from build123d import *

# Parameters (mm, degrees)
BOSS_EXTRUDE1_DEPTH     = 190
SKETCH2_W               = 50
SKETCH2_H               = 20
CUT_EXTRUDE1_DEPTH      = 50
SKETCH3_W               = 50
SKETCH3_H               = 80
CUT_EXTRUDE2_DEPTH      = 50
SKETCH4_W               = 50
SKETCH4_H               = 35
CUT_EXTRUDE4_DEPTH      = 50
SKETCH9_W               = 15
SKETCH9_H               = 5
BOSS_EXTRUDE4_DEPTH     = 5
SKETCH5_R               = 1
CUT_EXTRUDE5_DEPTH      = 10
CUT_EXTRUDE6_DEPTH      = 100
CUT_EXTRUDE6_DEPTH_BACK = 10
SKETCH6_R               = 1
FILLET1_R               = 1
FILLET2_R               = 2


with BuildPart() as part:
    # Sketch1 → Boss-Extrude1 (new body)
    with BuildSketch(Plane.XY):
        Polygon((-5.73630137, 0.530821918), (9.26369863, 0.530821918), (9.26369863, -1.469178082), (59.26369863, -1.469178082), (59.26369863, 0.530821918), (74.26369863, 0.530821918), (74.26369863, -4.469178082), (69.26369863, -4.469178082), (69.26369863, -7.469178082), (66.26369863, -7.469178082), (66.26369863, -4.469178082), (2.26369863, -4.469178082), (2.26369863, -7.469178082), (-0.73630137, -7.469178082), (-0.73630137, -4.469178082), (-5.73630137, -4.469178082), align=None)
    extrude(amount=BOSS_EXTRUDE1_DEPTH)

    # Sketch2 → Cut-Extrude1 (cut)
    with BuildSketch(Plane(origin=(0, -1.469178082, 0), x_dir=(1, 0, 0), z_dir=(0, 1, 0))):
        with Locations((34.26369863, -10)):
            Rectangle(SKETCH2_W, SKETCH2_H)
        with Locations((34.26369863, -190)):
            Rectangle(SKETCH2_W, SKETCH2_H)
    extrude(amount=-CUT_EXTRUDE1_DEPTH, mode=Mode.SUBTRACT)

    # Sketch3 → Cut-Extrude2 (cut)
    with BuildSketch(Plane(origin=(0, -1.469178082, 0), x_dir=(1, 0, 0), z_dir=(0, 1, 0))):
        with Locations((34.26369863, -75)):
            Rectangle(SKETCH3_W, SKETCH3_H)
    extrude(amount=-CUT_EXTRUDE2_DEPTH, mode=Mode.SUBTRACT)

    # Sketch4 → Cut-Extrude4 (cut)
    with BuildSketch(Plane(origin=(0, -1.469178082, 0), x_dir=(1, 0, 0), z_dir=(0, 1, 0))):
        with Locations((34.26369863, -147.5)):
            Rectangle(SKETCH4_W, SKETCH4_H)
    extrude(amount=-CUT_EXTRUDE4_DEPTH, mode=Mode.SUBTRACT)

    # Sketch9 → Boss-Extrude4 (add)
    with BuildSketch(Plane(origin=(0, 0, 0), x_dir=(-1, 0, 0), z_dir=(0, 0, -1))):
        with Locations((-66.76369863, -1.969178082)):
            Rectangle(SKETCH9_W, SKETCH9_H)
        with Locations((-1.76369863, -1.969178082)):
            Rectangle(SKETCH9_W, SKETCH9_H)
    extrude(amount=BOSS_EXTRUDE4_DEPTH)

    # Sketch5 → Cut-Extrude5 (cut)
    with BuildSketch(Plane(origin=(0, -4.469178082, 0), x_dir=(-1, 0, 0), z_dir=(0, -1, 0))):
        with Locations(Location((-71.76369863, -162.5, 0), (0, 0, 90))):
            Circle(SKETCH5_R)
        with Locations(Location((3.23630137, -162.5, 0), (0, 0, 90))):
            Circle(SKETCH5_R)
    extrude(amount=-CUT_EXTRUDE5_DEPTH, mode=Mode.SUBTRACT)

    # Sketch6 → Cut-Extrude6 (cut, two sides: drawn at the far end of the back side and taken through both)
    with BuildSketch(Plane(origin=(0, -4.469178082, 0), x_dir=(-1, 0, 0), z_dir=(0, -1, 0)).offset(-CUT_EXTRUDE6_DEPTH_BACK)):
        with Locations(Location((3.23630137, -87.5, 0), (0, 0, 270))):
            Circle(SKETCH6_R)
        with Locations(Location((3.23630137, -17.5, 0), (0, 0, 270))):
            Circle(SKETCH6_R)
        with Locations(Location((-71.76369863, -17.5, 0), (0, 0, 270))):
            Circle(SKETCH6_R)
        with Locations(Location((-71.76369863, -87.5, 0), (0, 0, 270))):
            Circle(SKETCH6_R)
    extrude(amount=CUT_EXTRUDE6_DEPTH + CUT_EXTRUDE6_DEPTH_BACK, mode=Mode.SUBTRACT)

    # Fillet1
    fillet1_edges = [part.edges().sort_by_distance(p)[0] for p in [
        (9.26369863, -2.969178082, 165),
        (59.26369863, -2.969178082, 130),
        (9.26369863, -2.969178082, 130),
        (59.26369863, -2.969178082, 165),
        (69.26369863, -4.469178082, 95),
        (66.26369863, -4.469178082, 95),
        (2.26369863, -4.469178082, 95),
        (-0.73630137, -4.469178082, 95),
        (59.26369863, -2.969178082, 20),
        (9.26369863, -2.969178082, 20),
        (9.26369863, -2.969178082, 180),
        (59.26369863, -2.969178082, 180),
        (9.26369863, -2.969178082, 115),
        (59.26369863, -2.969178082, 35),
        (9.26369863, -2.969178082, 35),
        (59.26369863, -2.969178082, 115),
    ]]
    fillet(fillet1_edges, radius=FILLET1_R)

    # Fillet2
    fillet2_edges = [part.edges().sort_by_distance(p)[0] for p in [
        (59.26369863, -1.469178082, 27.5),
        (9.26369863, -1.469178082, 27.5),
        (9.26369863, -1.469178082, 172.5),
        (59.26369863, -1.469178082, 172.5),
        (59.26369863, -1.469178082, 122.5),
        (9.26369863, -1.469178082, 122.5),
    ]]
    fillet(fillet2_edges, radius=FILLET2_R - 0.0001)  # a hair under: the kernel refuses the full size


solid = part.part
CAD build for the part. Positions are in the model's coordinates, mm. A direction names the side the tool comes from. Coordinates: 2 decimals unless noted, no trailing zeros. Write each loop counter-clockwise with the first axis right and the second up, starting at its lowest first coordinate (ties: lowest second). Pieces come first, ordered by that corner, then holes. Notation, with made-up numbers: M 66.25,-3.5 L 124.25,-3.5 A21 ccw 124.25,35.5 Z; hole C -19.5,4.25 d9. An arc over 180 degrees is marked long. Answer as a JSON object with one key per item and string values. Group by question number.
1) Mould opens along Z. For faces 1 (the face through (-5.736, -2, 94)), 2 (the face through (2, -2, -5)), 3 (the face through (34, -3, 115)), 4 (the face through (59.264, -2, 94)) say: +Z half, -Z half, draft (parallel to the pull), parting line (faces both ways), or undercut.
2) Saw through at D-D (y = -3.25). Give the number of separate pieces and of enclosed holes in the cut face, plus the area to 3 significant figures.
3) Saw through at A-A (z = 80.5). Write the cut outline in (x, y), plus the area to 3 significant figures.
4) Pin check, flat tips, straight feed: pin 1 Ø4.5 at (x, z) = (38.5, 27.5) entering from +Y; pin 2 Ø1 at (x, y) = (17.5, -2) entering from -Z; pin 3 Ø1.6 at (x, y) = (43.5, -3) entering from +Z; pin 4 Ø1 at (x, y) = (50.5, -0.5) entering from -Z. Stop position of each tip, or through.
5) Tool access for faces 5 (the face through (34, -1.469, 27)), 6 (the face through (9.264, -2, 91)), 7 (the face through (34, -3, 20)): list every direction of +Z, -Z, +X, -X, +Y, -Y with a clear straight run to the whole face (end or side of a thin tool).
6) Saw through at B-B (x = 54.5). Write the cut outline in (y, z), plus the area to 3 significant figures.
7) Wall check: line 1 (X direction, y = -1.7, z = 87.5); line 2 (Z direction, x = 51, y = -3.75); line 3 (X direction, y = -3.25, z = 64.5). Give the ranges that are in metal, low to high. Write a range as from..to.
Values follow:
{
 "1": {"face 1": "draft", "face 2": "-Z half", "face 3": "undercut", "face 4": "undercut"},
 "2": {"separate pieces": "1", "enclosed holes": "8", "area": "8,080 mm2"},
 "3": {"outline": "M -5.74,-4.47 L -1.74,-4.47 A1 cw -0.74,-5.47 L -0.74,-7.47 L 2.26,-7.47 L 2.26,-5.47 A1 cw 3.26,-4.47 L 9.26,-4.47 L 9.26,0.53 L -5.74,0.53 Z; M 59.26,-4.47 L 65.26,-4.47 A1 cw 66.26,-5.47 L 66.26,-7.47 L 69.26,-7.47 L 69.26,-5.47 A1 cw 70.26,-4.47 L 74.26,-4.47 L 74.26,0.53 L 59.26,0.53 Z", "area": "169 mm2"},
 "4": {"pin 1": "stops at y = -1.47", "pin 2": "stops at z = 20", "pin 3": "stops at z = 180", "pin 4": "passes through"},
 "5": {"face 5": "+Z, -Z, +Y", "face 6": "+Y, -Y", "face 7": "-Z, +Y, -Y"},
 "6": {"outline": "M -4.47,20 L -1.47,20 L -1.47,35 L -4.47,35 Z; M -4.47,115 L -1.47,115 L -1.47,130 L -4.47,130 Z; M -4.47,165 L -1.47,165 L -1.47,180 L -4.47,180 Z", "area": "135 mm2"},
 "7": {"line 1": "x = -5.74..-4.24, -2.24..9.26, 59.26..70.76, 72.76..74.26", "line 2": "z = 20..35, 115..130, 165..180", "line 3": "x = -5.74..9.26, 59.26..74.26"}
}
